The listing builds one solid part. Answer for the finished solid, in the listing's coordinates (mm). A direction names the side the tool comes from. Round coordinates to 2 decimals unless told otherwise and drop trailing zeros. Order: outer loops, then holes, each group sorted by start corner. A loop starts at its lowest first (then second) coordinate and runs counter-clockwise, first axis right, second up. Notation, with made-up numbers: (26.25, 63.5) -> (74.25, 63.5) arc R19 ccw to (74.25, 83.5) -> close; hole circle Ø10 at (88.25, 68). An arc over 180 degrees is marked (long way). Answer in a Markdown table with one row per item. Add a question column.
```python
from build123d import *

# Parameters (mm, degrees)
SKETCH002_R             = 33.5
PAD002_DEPTH            = 26
SKETCH003_R             = 12.5
PAD003_DEPTH            = 60
PAD004_DEPTH            = 12.5
POCKET_DEPTH            = 10
SKETCH024_R             = 2
POCKET007_DEPTH         = 2
BODY002_PLACEMENT_ANGLE = 270


with BuildPart() as part:
    # Sketch002 → Pad002 (new body)
    with BuildSketch(Plane.YZ):
        Circle(SKETCH002_R)
    extrude(amount=PAD002_DEPTH)

    # Sketch003 → Pad003 (join)
    with BuildSketch(Plane.YZ):
        Circle(SKETCH003_R)
    extrude(amount=-PAD003_DEPTH)

    # Sketch004 → Pad004 (join, symmetric)
    with BuildSketch(Plane.XZ):
        Polygon((-6, 12.5), (-6, -20), (-37, -20), (-37, -18), (-8, -18), (-8, 12.5), align=None)
    extrude(amount=PAD004_DEPTH, both=True)

    # Sketch005 → Pocket (cut)
    with BuildSketch(Plane.YZ):
        with BuildLine():
            ThreePointArc((12.5, 0), (0, 12.5), (-12.5, 0))
            Line((-13.5, 0), (-12.5, 0))
            Line((-13.5, 13.5), (-13.5, 0))
            Line((13.5, 13.5), (-13.5, 13.5))
            Line((13.5, 0), (13.5, 13.5))
            Line((12.5, 0), (13.5, 0))
        make_face()
    extrude(amount=-POCKET_DEPTH, mode=Mode.SUBTRACT)

    # Sketch024 (on Face11 of Pocket) → Pocket007 (cut)
    with BuildSketch(Plane.YX.offset(20)):
        with Locations((8, -15.5)):
            Circle(SKETCH024_R)
        with Locations((-8, -15.5)):
            Circle(SKETCH024_R)
        with Locations((-8, -29.5)):
            Circle(SKETCH024_R)
        with Locations((8, -29.5)):
            Circle(SKETCH024_R)
    extrude(amount=-POCKET007_DEPTH, mode=Mode.SUBTRACT)


with BuildPart() as part_1:
    # Body002 placement: moved
    add(part.part.moved(Location((-87, -84.5, 25))).rotate(Axis((-87, -84.5, 25), (0, 0, 1)), BODY002_PLACEMENT_ANGLE))


solid = part_1.part
```
Item 1: The part is cut by section B-B, the plane x = -87. Give the vertices of the cut face in (y, z).
Item 2: Find the intervals of material crossed by probe 1 along Y at (x, z) = (-95, 5.65); probe 2 along Y at (x, z) = (-89, -5); probe 3 along Z at (x, y) = (-76.5, -105.5), in increasing order. Write a range as [from, to].
Item 3: The part is cut by section C-C, the plane x = -79. Give the vertices of the cut face in (y, z), and give its area (3 significant figures).
Item 4: Flat-ended cylindrical pins translate along their axes: P1, Ø16, axis at y = -66, z = 14.5, coming from the -X side; P2, Ø12, axis at x = -78, z = 47, coming from the +Y side; P3, Ø1, axis at x = -84, z = 6, coming from the +Y side; P4, Ø12, axis at x = -67, y = -55.5, coming from the +Z side. Find the tip coordinate at first contact, or state that the pin passes through.
Item 5: The part is cut by section D-D, the plane y = -36.5. Give the vertices of the cut face in (x, z).
Item 6: For a pull along X with two mould halves and no side action, classify faces 1 (the face through (-73, -84.5, 25)), 2 (the face through (-55.047, -97.318, 35.062)), 3 (the face through (-77.092, -69.601, 5.986)) as released by +X, released by -X, zero draft, split by the parting line, or undercut.
Item 7: The part is cut by section A-A, the plane y = -55. Give the vertices of the cut face in (x, z), and give its area (3 significant figures).
Item 8: A tool of negligible diameter and unlimited length cuts with its end or side. For faces 4 (the face through (-77.925, -56.686, 5.986)), 5 (the face through (-99.5, -69, 6)), 6 (the face through (-87, -62, 7)), 7 (the face through (-87, -47.5, 6)), from which of +Z, -Z, +X, -X, +Y, -Y can it reach the whole face along a straight path? Write none if from no direction.
Resolved:
| question | item | result |
|---|---|---|
| 1 | outline | (-110.5, -8.5) -> (-84.5, -8.5) -> (-84.5, 12.5) -> (-78.5, 12.5) -> (-78.5, 5) -> (-47.5, 5) -> (-47.5, 7) -> (-76.5, 7) -> (-76.5, 12.5) -> (-24.5, 12.5) -> (-24.5, 37.5) -> (-84.5, 37.5) -> (-84.5, 58.5) -> (-110.5, 58.5) -> close |
| 2 | probe 1 | [-110.5, -84.5], [-78.5, -71], [-67, -57], [-53, -47.5] |
| 2 | probe 2 | [-110.5, -84.5] |
| 2 | probe 3 | [-6.81, 56.81] |
| 3 | outline | (-110.5, -7.53) -> (-84.5, -7.53) -> (-84.5, 15.4) -> (-78.5, 15.4) -> (-78.5, 5) -> (-71, 5) -> (-71, 7) -> (-76.5, 7) -> (-76.5, 15.4) -> (-24.5, 15.4) -> (-24.5, 34.6) -> (-84.5, 34.6) -> (-84.5, 57.53) -> (-110.5, 57.53) -> close; (-67, 5) -> (-57, 5) -> (-57, 7) -> (-67, 7) -> close; (-53, 5) -> (-47.5, 5) -> (-47.5, 7) -> (-53, 7) -> close |
| 3 | area | 2,910 mm2 |
| 4 | P1 | x = -99.5 |
| 4 | P2 | y = -84.5 |
| 4 | P3 | y = -47.5 |
| 4 | P4 | through |
| 5 | outline | circle Ø25 at (-87, 25) |
| 6 | face 1 | zero draft |
| 6 | face 2 | split by the parting line |
| 6 | face 3 | undercut |
| 7 | outline | (-99.5, 5) -> (-97, 5) -> (-97, 7) -> (-99.5, 7) -> close; circle Ø25 at (-87, 25); (-93, 5) -> (-81, 5) -> (-81, 7) -> (-93, 7) -> close; (-77, 5) -> (-74.5, 5) -> (-74.5, 7) -> (-77, 7) -> close |
| 7 | area | 525 mm2 |
| 8 | face 4 | -Z |
| 8 | face 5 | +Z, -Z, -X, +Y |
| 8 | face 6 | +X, -X, +Y |
| 8 | face 7 | -Z, +X, -X, +Y |
